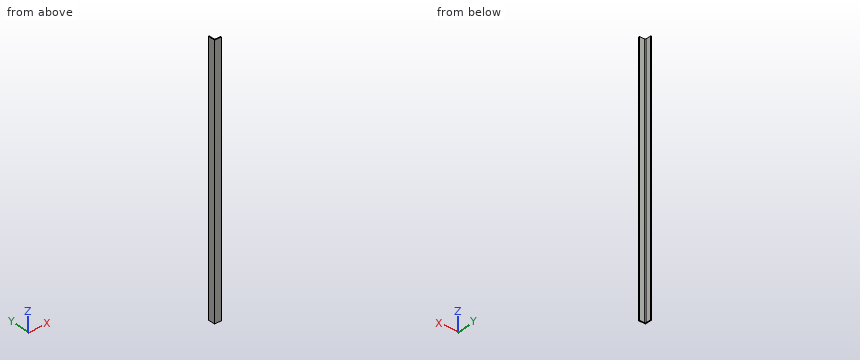
Autodesk Inventor part; units mm, degrees
ref_plane "Plano inicial" through (0, 0, 0) normal (0, 0, 1) x (1, 0, 0)
ref_plane "Plano final" through (0, 0, 1401) normal (0, 0, 1) x (1, 0, 0)
ref_plane "YZ Plane" through (0, 0, 0) normal (1, 0, 0) x (0, 1, 0)
ref_plane "Plano inicial" through (0, 0, 0) normal (0, 0, 1) x (1, 0, 0)
ref_plane "Plano final" through (0, 0, 1401) normal (0, 0, 1) x (1, 0, 0)
sketch "Boceto" plane through (0, 0, 0) normal (0, 0, 1) x (1, 0, 0)
  line L0 (38.1, 0) -> (0, 0)
  line L1 (0, 0) -> (0, 38.1)
  line L2 (0, 38.1) -> (2.4765, 38.1)
  line L3 (4.7625, 35.814) -> (4.7625, 9.5885)
  line L4 (9.5885, 4.7625) -> (35.814, 4.7625)
  line L5 (38.1, 2.4765) -> (38.1, 0)
  line L6 (0, -11.0414) -> (0, 31.5385) construction
  line L7 (-11.0414, 0) -> (31.5385, 0) construction
  arc A0 (4.7625, 9.5885) -> (9.5885, 4.7625) centre (9.5885, 9.5885) ccw
  arc A1 (4.7625, 35.814) -> (2.4765, 38.1) centre (2.4765, 35.814) ccw
  arc A2 (38.1, 2.4765) -> (35.814, 4.7625) centre (35.814, 2.4765) ccw
  line L8 (0, 48.4964) -> (0, -20.9644) construction
  line L9 (-20.9644, 0) -> (48.4964, 0) construction
  point P0 (4.7625, 38.1)
  point P1 (4.7625, 4.7625)
  point P2 (38.1, 4.7625)
  dimension "d0" = 38.1
  dimension "d1" = 38.1
  dimension "d2" = 4.7625
  dimension "d3" = 4.7625
  dimension "d10" = 0
  dimension "d11" = 0
  dimension "d14" = 4.826
  dimension "d15" = 2.286
extrude "Cuerpo" add sketch "Boceto" along normal up to surface (1401 mm away) from surface at 0
sketch "Sketch3" plane through (0, 0, 0) normal (0, 0, 1) x (1, 0, 0)
  line L0 (0, 0) -> (10, 0)
ref_plane "Work Plane3" through (0, 0, 0) normal (0, -1, 0) x (1, 0, 0)
sketch "Sketch4" plane through (0, 0, 0) normal (0, -1, 0) x (1, 0, 0)
  line L0 (-2, 0) -> (12, 0)
  line L1 (-2, 1401) -> (12, 1401)
  dimension "d17" = 1401
equation "\"d0\" = G_H"
equation "\"d1\" = G_H"
equation "\"d2\" = G_T"
equation "\"d3\" = G_T"
equation "\"d14\" = G_IR"
equation "\"d15\" = G_ER"
equation "\"d4\" = G_L"
equation "\"G_H\" = 38.1"
equation "\"G_T\" = 4.7625"
equation "\"G_ER\" = 2.286"
equation "\"G_IR\" = 4.826"
equation "\"G_L\" = d17"
equation "\"ex\" = 0"
equation "\"G_OFFSET_START\" = 0"
equation "\"G_OFFSET_END\" = 0"
equation "\"d13\" = G_OFFSET_END + B_L"
equation "\"B_L\" = 1401"
properties part number "AISC - L 1,5 x 1,5 x 3/16 - 55,157" material "Acero, suave"
The model under review builds one solid part; all positions refer to its coordinate system, in mm. Coordinates: 2 decimals unless noted, no trailing zeros. Write each loop counter-clockwise with the first axis right and the second up, starting at its lowest first coordinate (ties: lowest second). Pieces come first, ordered by that corner, then holes. Notation, with made-up numbers: (1.5, 39.5) - (46.5, 39.5) arc R11 cw to (46.5, 53.5) - close; hole circle Ø10 at (31, 61). An arc over 180 degrees is marked (long way). Write item = value, one per line.
(1) For line 1 (Y direction, x = 31, z = 416); line 2 (Y direction, x = 3.5, z = 998), list the stretches that pass through material, from the lowest coordinate up. Write a range as [from, to].
Result sheet:
line_1 = [0, 4.76]
line_2 = [0, 37.86]
(2) Consider section A-A, the plane z = 374. Give the boundary of the cut face in (x, y), then the cut area to 3 significant figures.
Result sheet:
outline = (0, 0) - (38.1, 0) - (38.1, 2.48) arc R2.29 ccw to (35.81, 4.76) - (9.59, 4.76) arc R4.83 cw to (4.76, 9.59) - (4.76, 35.81) arc R2.29 ccw to (2.48, 38.1) - (0, 38.1) - close
area = 343 mm^2
(3) Consider section B-B, the plane y = 29.5. Give the boundary of the cut face in (x, z).
Result sheet:
outline = (0, 0) - (4.76, 0) - (4.76, 1401) - (0, 1401) - close
(4) For P1, Ø13, axis at x = 27, z = 1026, coming from the +Y side; P2, Ø13, axis at y = 29, z = 397.5, coming from the +X side; P3, Ø10, axis at x = 15.5, y = 14, coming from the -Z side, all flat-tipped, find the tip position at first contact; note any pin that passes through.
Result sheet:
P1 = 4.76
P2 = 4.76
P3 = through
